Geometry check sheet. Reference: drawing and pictorial views, mm from the part's lowest x, y, z. A direction names the side the tool comes from. Round coordinates to 2 decimals unless told otherwise and drop trailing zeros. Order: outer loops, then holes, each group sorted by start corner. A loop starts at its lowest first (then second) coordinate and runs counter-clockwise, first axis right, second up.
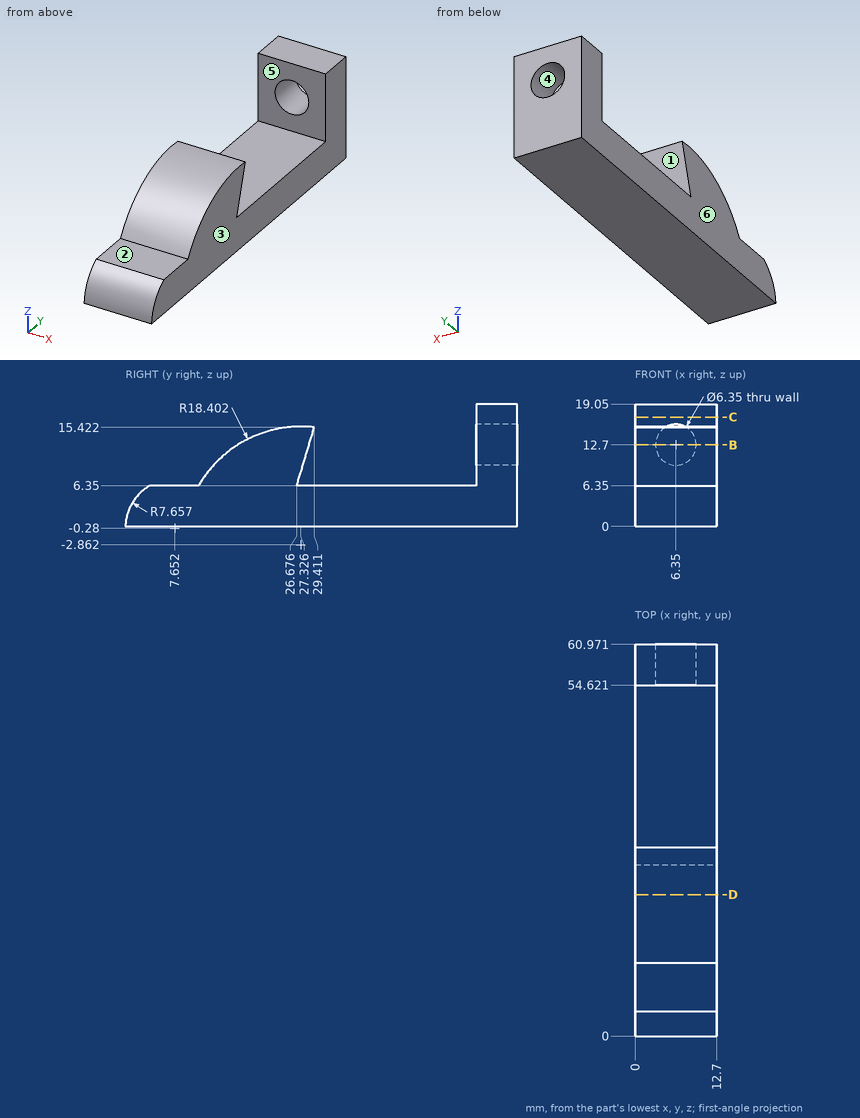
1) Scan lines: probe 1 along Y at (x, z) = (10.25, 12.75) (1 decimal); probe 2 along Y at (x, z) = (2.75, 11) (1 decimal); probe 3 along Y at (x, z) = (3, 18). Record each from-to range of solid material in increasing order.
2) Sectioned sample at B-B on z = 12.7. Record the cut outline in (x, y) (1 decimal), then the cut area to 3 significant figures.
3) Sectioned sample at D-D on y = 22. Record the cut outline in (x, z), then the cut area to 3 significant figures.
4) Go/stop test with flat-tipped pins: pin 1 Ø3 at (x, z) = (3, 7.5) entering from -Y; pin 2 Ø2 at (x, y) = (11, 38) entering from +Z; pin 3 Ø2.5 at (x, y) = (3.5, 8) entering from +Z; pin 4 Ø6 at (y, z) = (45, 12) entering from +X. Record where each tip stops, or that it passes through.
5) Draft check along Z on the marked faces 1, 2 and 3. Enter one of: released by +Z, released by -Z, zero draft, split by the parting line, or undercut.
6) Sectioned sample at C-C on z = 17. Record the cut outline in (x, y).
7) Tool access check on the marked faces 4, 5 and 6. Record the directions out of +Z, -Z, +X, -X, +Y, -Y that give a thin tool (end or side, any length) a straight path to the whole face; none if there is none.
Returned:
1. probe 1: y = 17.6 to 28.6, 54.6 to 61
1. probe 2: y = 15.2 to 28.1, 54.6 to 61
1. probe 3: y = 54.62 to 60.97
2. outline: (0, 17.5) - (12.7, 17.5) - (12.7, 28.6) - (0, 28.6) - close; (0, 54.6) - (3.2, 54.6) - (3.2, 61) - (0, 61) - close; (9.5, 54.6) - (12.7, 54.6) - (12.7, 61) - (9.5, 61) - close
2. area: 181 mm2
3. outline: (0, 0) - (12.7, 0) - (12.7, 14.75) - (0, 14.75) - close
3. area: 187 mm2
4. pin 1: stops at y = 3.27
4. pin 2: stops at z = 6.35
4. pin 3: stops at z = 6.35
4. pin 4: passes through
5. face 1: undercut
5. face 2: released by +Z
5. face 3: zero draft
6. outline: (0, 54.62) - (12.7, 54.62) - (12.7, 60.97) - (0, 60.97) - close
7. face 4: +Y
7. face 5: +Z, +X, -X
7. face 6: +Z, -Z, -X, +Y, -Y
